Build history of the part. All positions in model axes, mm. Face numbers are marked on the shaded views. A direction names the side the tool comes from. Round coordinates to 2 decimals unless told otherwise and drop trailing zeros. Loops run counter-clockwise (first coordinate to the right, second up) from the corner with the lowest first, then second, coordinate; pieces in that order, holes last. Notation, with made-up numbers: (-19, 41.25) - (28, 41.25) arc R32 cw to (28, 73.25) - close; hole circle Ø5 at (25, -26.5). An arc over 180 degrees is marked (long way). Use a Markdown table: item, result.
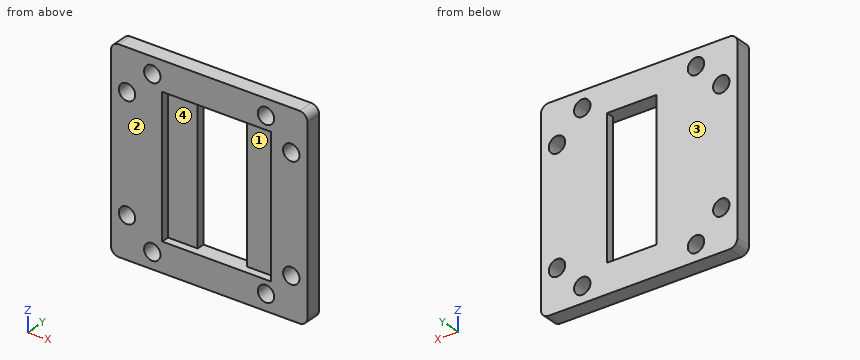
Autodesk Inventor part; units mm, degrees
ref_plane "Work Plane1" through (124.725, 49.8, -24.875) normal (0, 1, 0) x (0, 0, 1)
ref_plane "YZ Plane" through (0, 0, 0) normal (1, 0, 0) x (0, 1, 0)
ref_plane "XZ Plane" through (0, 0, 0) normal (0, 1, 0) x (-1, 0, 0)
sketch "Sketch1" plane through (0, 0, 0) normal (0, 1, 0) x (-1, 0, 0)
  line L0 (-155.225, -15) -> (-155.225, 15)
  line L1 (-155.225, 15) -> (-147.725, 15)
  line L2 (-147.725, 15) -> (-147.725, -15)
  line L3 (-147.725, -15) -> (-155.225, -15)
  circle A0 centre (-171.5, -21.9) radius 1.875
  circle A1 centre (-127.7, 21.9) radius 1.875
  circle A2 centre (-127.7, -21.9) radius 1.875
  circle A3 centre (-171.5, 21.9) radius 1.875
  circle A4 centre (-135.2, 20.8) radius 2.0734
  circle A5 centre (-164, -20.8) radius 2.0734
  circle A6 centre (-135.2, -20.8) radius 2.0734
  circle A7 centre (-128.8, -14.4) radius 2.0734
  circle A8 centre (-128.8, 14.4) radius 2.0734
  circle A9 centre (-164, 20.8) radius 2.0734
  circle A10 centre (-170.4, -14.4) radius 2.0734
  circle A11 centre (-170.4, 14.4) radius 2.0734
  line L4 (-172.5, 24.875) -> (-126.7, 24.875)
  arc A12 (-172.5, 24.875) -> (-174.475, 22.9) centre (-172.5, 22.9) ccw
  line L5 (-174.475, -22.9) -> (-174.475, 22.9)
  arc A13 (-174.475, -22.9) -> (-172.5, -24.875) centre (-172.5, -22.9) ccw
  line L6 (-126.7, -24.875) -> (-172.5, -24.875)
  arc A14 (-126.7, -24.875) -> (-124.725, -22.9) centre (-126.7, -22.9) ccw
  line L7 (-124.725, 22.9) -> (-124.725, -22.9)
  arc A15 (-124.725, 22.9) -> (-126.7, 24.875) centre (-126.7, 22.9) ccw
  point P0 (0, 0)
ref_plane "Work Plane1" through (124.725, 49.8, -24.875) normal (0, 1, 0) x (0, 0, 1)
extrude "Extrusion1" add sketch "Sketch1" along normal blind 4 from surface at 49.8 contours A0 | A1 | A2 | A3 | L4 A15 L7 A14 L6 A13 L5 A12
sketch "Sketch2" plane through (126.7, 53.8, -24.875) normal (0, 1, 0) x (1, 0, 0)
  line L0 (28.525, -9.875) -> (21.025, -9.875)
  line L1 (28.525, -39.875) -> (28.525, -9.875)
  line L2 (21.025, -39.875) -> (28.525, -39.875)
  line L3 (21.025, -9.875) -> (21.025, -39.875)
  circle A0 centre (8.5, -45.675) radius 2.0734
  circle A1 centre (37.3, -4.075) radius 2.0734
  circle A2 centre (8.5, -4.075) radius 2.0734
  circle A3 centre (2.1, -10.475) radius 2.0734
  circle A4 centre (2.1, -39.275) radius 2.0734
  circle A5 centre (37.3, -45.675) radius 2.0734
  circle A6 centre (43.7, -10.475) radius 2.0734
  circle A7 centre (43.7, -39.275) radius 2.0734
  arc A8 (47.775, -1.975) -> (45.8, 0) centre (45.8, -1.975) ccw
  line L4 (0, 0) -> (45.8, 0)
  arc A9 (0, 0) -> (-1.975, -1.975) centre (0, -1.975) ccw
  line L5 (-1.975, -47.775) -> (-1.975, -1.975)
  arc A10 (-1.975, -47.775) -> (0, -49.75) centre (0, -47.775) ccw
  line L6 (45.8, -49.75) -> (0, -49.75)
  arc A11 (45.8, -49.75) -> (47.775, -47.775) centre (45.8, -47.775) ccw
  line L7 (47.775, -1.975) -> (47.775, -47.775)
  line L8 (18.525, -42.375) -> (31.025, -42.375)
  line L9 (31.025, -42.375) -> (31.025, -7.375)
  line L10 (31.025, -7.375) -> (18.525, -7.375)
  line L11 (18.525, -7.375) -> (18.525, -42.375)
  line L12 (45.8, 0) -> (50.05, 0)
  line L13 (50.05, 0) -> (50.05, -49.75)
  line L14 (50.05, -49.75) -> (45.8, -49.75)
  line L15 (45.8, -49.75) -> (45.8, 0)
  line L16 (50.05, -49.75) -> (47.925, -49.75)
  line L17 (47.925, -49.75) -> (47.925, 0)
  line L18 (47.925, 0) -> (50.05, 0)
  line L19 (50.05, 0) -> (50.05, -49.75)
  arc A12 (45.8, -49.875) -> (47.9, -47.775) centre (45.8, -47.775) ccw
  line L20 (45.8, -49.875) -> (0, -49.875)
  arc A13 (-2.1, -47.775) -> (0, -49.875) centre (0, -47.775) ccw
  line L21 (-2.1, -47.775) -> (-2.1, -1.975)
  arc A14 (0, 0.125) -> (-2.1, -1.975) centre (0, -1.975) ccw
  line L22 (0, 0.125) -> (45.8, 0.125)
  arc A15 (47.9, -1.975) -> (45.8, 0.125) centre (45.8, -1.975) ccw
  line L23 (47.9, -1.975) -> (47.9, -47.775)
  line L24 (18.525, -42.375) -> (11.025, -42.375)
  line L25 (11.025, -42.375) -> (11.025, -7.375)
  line L26 (11.025, -7.375) -> (18.525, -7.375)
  line L27 (18.525, -7.375) -> (18.525, -42.375)
  line L28 (31.025, -42.375) -> (38.525, -42.375)
  line L29 (38.525, -42.375) -> (38.525, -7.375)
  line L30 (38.525, -7.375) -> (31.025, -7.375)
  line L31 (31.025, -7.375) -> (31.025, -42.375)
  point P0 (-126.7, -24.875)
  point P1 (47.925, -49.75)
  point P2 (46.5137, -49.75)
  point P3 (46.5137, 0)
  point P4 (31.025, -7.375)
  point P5 (18.525, -7.375)
  dimension "d2" = 2.5
  dimension "d3" = 4.25
  dimension "d4" = 2.125
  dimension "d15" = 0.125
  dimension "d16" = 7.5
  dimension "d17" = 7.5
extrude "Extrusion2" cut sketch "Sketch2" against normal up to surface (4 mm away) contours L11 L10 L9 L8
extrude "Extrusion3" [suppressed]
extrude "Extrusion4" [suppressed]
fillet "Fillet1" [suppressed]
sketch "Sketch3" plane through (176.75, 51.8, 22.875) normal (1, 0, 0) x (0, 0, -1)
  line L0 (7.875, -21.425) -> (7.875, -28.925)
  line L1 (7.875, -28.925) -> (37.875, -28.925)
  line L2 (37.875, -28.925) -> (37.875, -21.425)
  line L3 (37.875, -21.425) -> (7.875, -21.425)
  line L4 (5.825, -9.7) -> (39.925, -9.7)
  line L5 (39.925, -44.1) -> (39.925, -9.7)
  line L6 (5.825, -44.1) -> (39.925, -44.1)
  line L7 (5.825, -9.7) -> (5.825, -44.1)
  line L8 (2.875, -16.425) -> (2.875, -33.925)
  line L9 (2.875, -33.925) -> (42.875, -33.925)
  line L10 (42.875, -33.925) -> (42.875, -16.425)
  line L11 (42.875, -16.425) -> (2.875, -16.425)
  point P0 (22.875, -51.8)
  dimension "d12" = 5
extrude "Extrusion5" [suppressed]
extrude "Extrusion6" cut sketch "Sketch2" along normal blind 2 from surface at -4 contours L24 L25 L26 L11 | L9 L30 L29 L28
properties part number "Lens Top Light Cover"
Q1. Pull direction Z, two halves, no side cores. Call the marked faces 1 and 2: pulls with the +Z half, pulls with the -Z half, needs draft (parallel to the pull), parting line crosses it, or undercut.
Results found:
| item | result |
|---|---|
| face 1 | undercut |
| face 2 | needs draft |
Q2. Cut at C-C, the plane x = 164. List the corners of the cut face in (y, z) (3 decimals), plus the area to 3 significant figures.
Results found:
| item | result |
|---|---|
| outline | (49.8, -24.875) - (53.8, -24.875) - (53.8, -22.873) - (49.8, -22.873) - close; (49.8, -18.727) - (53.8, -18.727) - (53.8, 18.727) - (49.8, 18.727) - (49.8, 17.5) - (51.8, 17.5) - (51.8, -17.5) - (49.8, -17.5) - close; (49.8, 22.873) - (53.8, 22.873) - (53.8, 24.875) - (49.8, 24.875) - close |
| area | 95.8 mm2 |
Q3. Drop flat-ended pins along their axis: pin 1 (2.5 mm diameter, centred on x = 128.8, z = -14.4, fed in from -Y); pin 2 (6 mm diameter, centred on x = 162, z = 5, fed in from -Y). Give the stop position or say it passes through.
Results found:
| item | result |
|---|---|
| pin 1 | passes through |
| pin 2 | stops at y = 51.8 |
Q4. Cut at B-B, the plane y = 50.4. Count the separate pieces of the cut face and the enclosed holes in it, plus the area to 3 significant figures.
Results found:
| item | result |
|---|---|
| separate pieces | 1 |
| enclosed holes | 9 |
| area | 1,400 mm2 |
Q5. Cut at A-A, the plane x = 148.5. List the corners of the cut face in (y, z) (3 decimals).
Results found:
| item | result |
|---|---|
| outline | (49.8, -24.875) - (53.8, -24.875) - (53.8, -17.5) - (49.8, -17.5) - close; (49.8, 17.5) - (53.8, 17.5) - (53.8, 24.875) - (49.8, 24.875) - close |
Q6. Which spindle directions (+Z, -Z, +X, -X, +Y, -Y) get a long thin tool onto all of the face, cutting with end or side? Do the marked faces 3 and 4. Say none if no direction does.
Results found:
| item | result |
|---|---|
| face 3 | +Z, -Z, +X, -X, +Y |
| face 4 | -Y |
Q7. Cut at D-D, the plane z = 20.8. List the corners of the cut face in (x, y) (3 decimals), plus the area to 3 significant figures.
Results found:
| item | result |
|---|---|
| outline | (124.725, 49.8) - (133.127, 49.8) - (133.127, 53.8) - (124.725, 53.8) - close; (137.273, 49.8) - (161.927, 49.8) - (161.927, 53.8) - (137.273, 53.8) - close; (166.073, 49.8) - (174.475, 49.8) - (174.475, 53.8) - (166.073, 53.8) - close |
| area | 166 mm2 |
Q8. Probe line 1 (Z direction, x = 135.2, y = 52.2) (3 decimals); line 2 (Z direction, x = 128.8, y = 50.8) (3 decimals); line 3 (Z direction, x = 152, y = 51.35) (3 decimals). List the from-to ranges inside material, lowest first.
Results found:
| item | result |
|---|---|
| line 1 | z = -24.875 to -22.873, -18.727 to 18.727, 22.873 to 24.875 |
| line 2 | z = -24.875 to -16.473, -12.327 to 12.327, 16.473 to 24.875 |
| line 3 | z = -24.875 to -17.5, 17.5 to 24.875 |
